Here's the drawing with two shaded views (mm, measured from the low corner). I have some questions. A direction names the side the tool comes from. Round coordinates to 2 decimals unless told otherwise and drop trailing zeros. Loops run counter-clockwise (first coordinate to the right, second up) from the corner with the lowest first, then second, coordinate; pieces in that order, holes last.
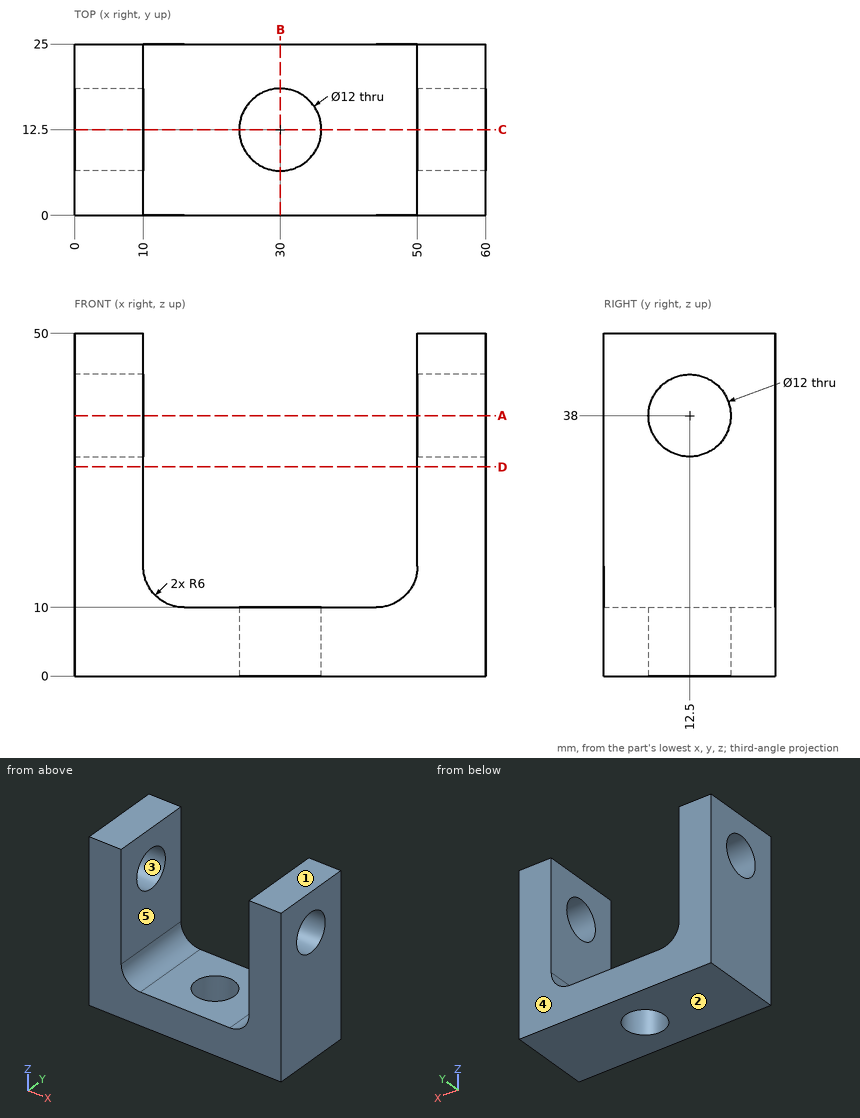
Item 1: If we section it at B-B, the plane x = 30: Please give me the cut outline in (y, z).
Results list:
outline: (0, 0) - (6.5, 0) - (6.5, 10) - (0, 10) - close; (18.5, 0) - (25, 0) - (25, 10) - (18.5, 10) - close
Item 2: If we section it at D-D, the plane z = 30.5: Please give me the cut outline in (x, y), then the cut area to 3 significant figures.
Results list:
outline: (0, 0) - (10, 0) - (10, 25) - (0, 25) - close; (50, 0) - (60, 0) - (60, 25) - (50, 25) - close
area: 500 mm2
Item 3: We'd pull the mould along Z, two halves only. Please class the marked faces 1, 2 and 3: released by +Z, released by -Z, zero draft, split by the parting line, or undercut.
Results list:
face 1: released by +Z
face 2: released by -Z
face 3: undercut
Item 4: For the marked faces 4 and 5, which set-ups out of +Z, -Z, +X, -X, +Y, -Y let a thin tool reach every point of the face, with its end or its side?
Results list:
face 4: +Z, -Z, +X, -X, +Y
face 5: +Z, +Y, -Y
Item 5: If we section it at C-C, the plane y = 12.5: Please give me the cut outline in (x, z).
Results list:
outline: (0, 0) - (24, 0) - (24, 10) - (16, 10) arc R6 cw to (10, 16) - (10, 32) - (0, 32) - close; (0, 44) - (10, 44) - (10, 50) - (0, 50) - close; (36, 0) - (60, 0) - (60, 32) - (50, 32) - (50, 16) arc R6 cw to (44, 10) - (36, 10) - close; (50, 44) - (60, 44) - (60, 50) - (50, 50) - close
Item 6: Will these pins go through, and if not, where does the flat tip stop? pin 1 (14 mm diameter, centred on y = 12.5, z = 38, fed in from -X); pin 2 (12 mm diameter, centred on x = 20, y = 13, fed in from +Z).
Results list:
pin 1: stops at x = 0
pin 2: stops at z = 10.34
Item 7: If we section it at A-A, the plane z = 38: Please give me the cut outline in (x, y).
Results list:
outline: (0, 0) - (10, 0) - (10, 6.5) - (0, 6.5) - close; (0, 18.5) - (10, 18.5) - (10, 25) - (0, 25) - close; (50, 0) - (60, 0) - (60, 6.5) - (50, 6.5) - close; (50, 18.5) - (60, 18.5) - (60, 25) - (50, 25) - close
Item 8: If I drill on line 1 along Y through (x, z) = (4.25, 38); line 2 along X through (y, z) = (10.25, 23); line 3 along Z through (x, y) = (54.75, 12.5), over which ranges is the centre line in solid material (lowest first)?
Results list:
line 1: y = 0 to 6.5, 18.5 to 25
line 2: x = 0 to 10, 50 to 60
line 3: z = 0 to 32, 44 to 50
